Verification items for this drawing (mm, ordinates from the low corner). A direction names the side the tool comes from. Round coordinates to 2 decimals unless told otherwise and drop trailing zeros. Loops run counter-clockwise (first coordinate to the right, second up) from the corner with the lowest first, then second, coordinate; pieces in that order, holes last. Notation, with made-up numbers: M -17.5,19.5 L 23.5,19.5 A24 ccw 23.5,49.5 Z; hole C 32,14 d6. An arc over 180 degrees is marked long. Answer in a Markdown table with one row per item. Add a question column.
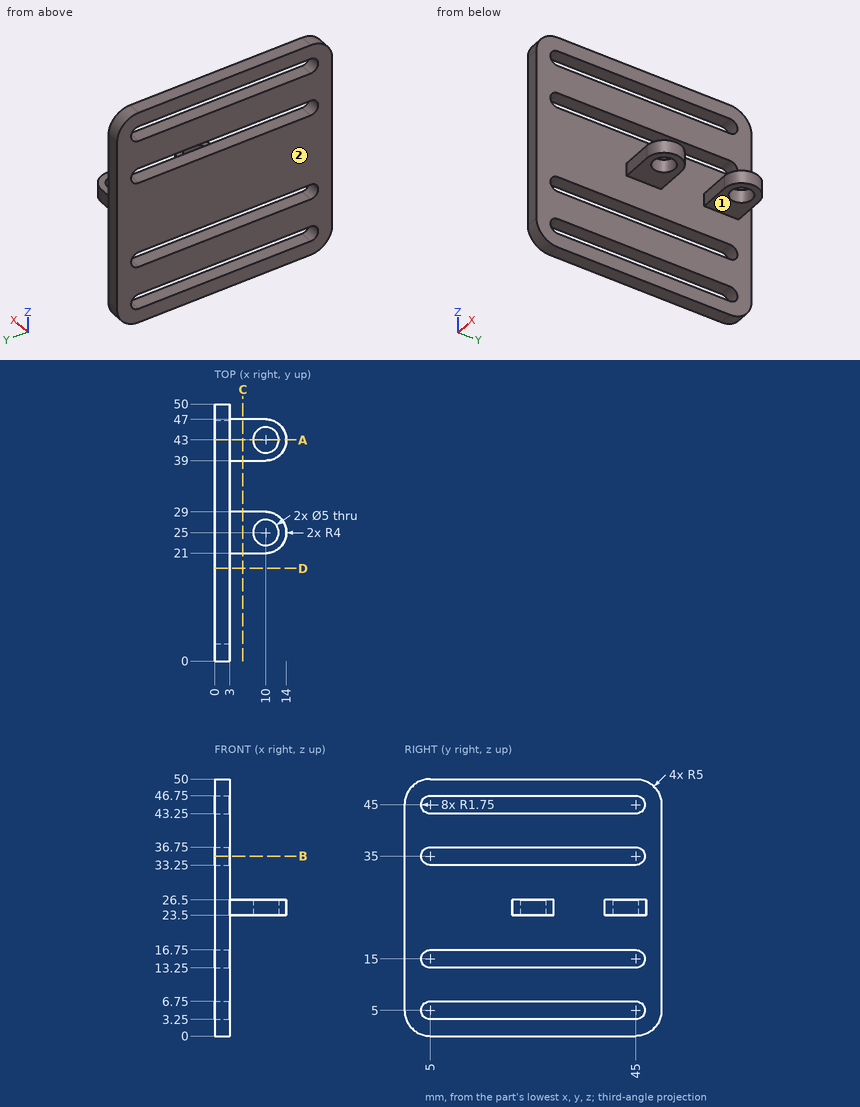
1) Cross-section at D-D, the plane y = 18. Record the boundary of the cut face in (x, z), plus the area to 3 significant figures.
2) Set-up check for the marked faces 1 and 2: record each of +Z, -Z, +X, -X, +Y, -Y from which the full face is reachable in a straight line by a thin tool's end or side.
3) Thickness scan on L1, parallel to Y at x = 10, z = 25.1; L2, parallel to Z at x = 1.75, y = 19; L3, parallel to Y at x = 7.75, z = 26. Record the ranges inside material, lowest first. Write a range as [from, to].
4) Cross-section at A-A, the plane y = 43. Record the boundary of the cut face in (x, z), plus the area to 3 significant figures.
5) Go/stop test with flat-tipped pins: pin 1 (0.9 mm diameter, centred on x = 8, z = 24.5, fed in from -Y); pin 2 (2.5 mm diameter, centred on x = 5.5, z = 25, fed in from +Y); pin 3 (4 mm diameter, centred on x = 9, y = 42, fed in from -Z). Record where each tip stops, or that it passes through.
6) Cross-section at B-B, the plane z = 35. Record the boundary of the cut face in (x, y), plus the area to 3 significant figures.
7) Cross-section at C-C, the plane x = 5.5. Record the boundary of the cut face in (y, z).
Worked answers:
| question | item | result |
|---|---|---|
| 1 | outline | M 0,0 L 3,0 L 3,3.25 L 0,3.25 Z; M 0,6.75 L 3,6.75 L 3,13.25 L 0,13.25 Z; M 0,16.75 L 3,16.75 L 3,33.25 L 0,33.25 Z; M 0,36.75 L 3,36.75 L 3,43.25 L 0,43.25 Z; M 0,46.75 L 3,46.75 L 3,50 L 0,50 Z |
| 1 | area | 108 mm2 |
| 2 | face 1 | -Z, +X, +Y, -Y |
| 2 | face 2 | +Z, -Z, -X, +Y, -Y |
| 3 | L1 | y = [21, 22.5], [27.5, 29], [39, 40.5], [45.5, 47] |
| 3 | L2 | z = [0, 3.25], [6.75, 13.25], [16.75, 33.25], [36.75, 43.25], [46.75, 50] |
| 3 | L3 | y = [21, 23.91], [26.09, 29], [39, 41.91], [44.09, 47] |
| 4 | outline | M 0,0 L 3,0 L 3,3.25 L 0,3.25 Z; M 0,6.75 L 3,6.75 L 3,13.25 L 0,13.25 Z; M 0,16.75 L 3,16.75 L 3,23.5 L 7.5,23.5 L 7.5,26.5 L 3,26.5 L 3,33.25 L 0,33.25 Z; M 0,36.75 L 3,36.75 L 3,43.25 L 0,43.25 Z; M 0,46.75 L 3,46.75 L 3,50 L 0,50 Z; M 12.5,23.5 L 14,23.5 L 14,26.5 L 12.5,26.5 Z |
| 4 | area | 126 mm2 |
| 5 | pin 1 | stops at y = 21 |
| 5 | pin 2 | stops at y = 47 |
| 5 | pin 3 | stops at z = 23.5 |
| 6 | outline | M 0,0 L 3,0 L 3,3.25 L 0,3.25 Z; M 0,46.75 L 3,46.75 L 3,50 L 0,50 Z |
| 6 | area | 19.5 mm2 |
| 7 | outline | M 21,23.5 L 29,23.5 L 29,26.5 L 21,26.5 Z; M 39,23.5 L 47,23.5 L 47,26.5 L 39,26.5 Z |
